Geometry check sheet. Reference: the model listing, model coordinates, mm. A direction names the side the tool comes from. Round coordinates to 2 decimals unless told otherwise and drop trailing zeros. Order: outer loops, then holes, each group sorted by start corner. A loop starts at its lowest first (then second) coordinate and runs counter-clockwise, first axis right, second up. Notation, with made-up numbers: (-9, 83) -> (-1, 83) arc R31 cw to (-1, 120) -> close; hole circle Ø3 at (34.25, -27.5). An arc over 180 degrees is marked (long way). Answer as a JSON object with one key per item and string values. Group by question number.
Solid Edge part; units mm, degrees
sketch "Sketch1" plane through (0, 0, 0) normal (0, -1, 0) x (1, 0, 0)
  line L0 (16.5, 0) -> (16.5, 15)
  line L1 (16.5, 15) -> (21, 15)
  line L2 (21, 15) -> (21, 21)
  line L3 (21, 21) -> (16.5, 21)
  line L4 (16.5, 21) -> (12, 19.7942)
  line L5 (12, 0) -> (12, 19.7942)
  line L6 (12, 0) -> (16.5, 0)
revolve "RevolvedProtrusion1" add sketch "Sketch1" angle 360 about axis through (0, 0, 0) along (0, 0, 1)
properties material "Brass, yellow brass"
Item 1: Sectioned sample at C-C, the plane z = 6. Enter the section's corners in (x, y), then the cut area to 3 significant figures.
Item 2: Depth check by flat-ended pin: pin 1 Ø10 at (x, y) = (0, -5) entering from -Z; pin 2 Ø1.5 at (y, z) = (-7.5, 6) entering from +X; pin 3 Ø3 at (x, z) = (12, 10.5) entering from +Y; pin 4 Ø1 at (y, z) = (3.5, 11.5) entering from +X (3 decimals). Enter the tip coordinate at first touch or a pass-through.
Item 3: Sectioned sample at D-D, the plane y = -18. Enter the section's corners in (x, z).
Item 4: Sectioned sample at A-A, the plane x = 0. Enter the section's corners in (y, z), then the cut area to 3 significant figures.
Item 5: Thickness scan on L1, parallel to Y at x = 0, z = 5.75; L2, parallel to X at y = -0.5, z = 5.5; L3, parallel to Y at x = -9, z = 17. Record the ranges inside material, lowest first.
Item 6: Set-up check for faces 4 (the flat face through (-13, -11, 21)), 5 (the flat face through (-13, -11, 15)): record each of +Z, -Z, +X, -X, +Y, -Y from which the full face is reachable in a straight line by a thin tool's end or side.
Item 7: Mould release check, pull along X, two halves, no side actions. Record for faces 1 (the cylindrical face through (20.03, 6.31, 18.04)), 2 (the flat face through (1.15, -12.15, 0)), 3 (the conical face through (-2.66, -11.99, 19.87)): pulls with the +X half, pulls with the -X half, needs draft (parallel to the pull), parting line crosses it, or undercut.
Result:
{
 "1": {"outline": "circle Ø33 at (0, 0); hole circle Ø24 at (0, 0)", "area": "403 mm2"},
 "2": {"pin 1": "passes through", "pin 2": "stops at x = 15.06", "pin 3": "stops at y = 12.73", "pin 4": "stops at x = 16.225"},
 "3": {"outline": "(-10.82, 15) -> (10.82, 15) -> (10.82, 21) -> (-10.82, 21) -> close"},
 "4": {"outline": "(-21, 15) -> (-16.5, 15) -> (-16.5, 0) -> (-12, 0) -> (-12, 19.79) -> (-16.5, 21) -> (-21, 21) -> close; (12, 0) -> (16.5, 0) -> (16.5, 15) -> (21, 15) -> (21, 21) -> (16.5, 21) -> (12, 19.79) -> close", "area": "238 mm2"},
 "5": {"L1": "y = -16.5 to -12, 12 to 16.5", "L2": "x = -16.49 to -11.99, 11.99 to 16.49", "L3": "y = -18.97 to -7.94, 7.94 to 18.97"},
 "6": {"face 4": "+Z, +X, -X, +Y, -Y", "face 5": "-Z"},
 "7": {"face 1": "parting line crosses it", "face 2": "needs draft", "face 3": "undercut"}
}
